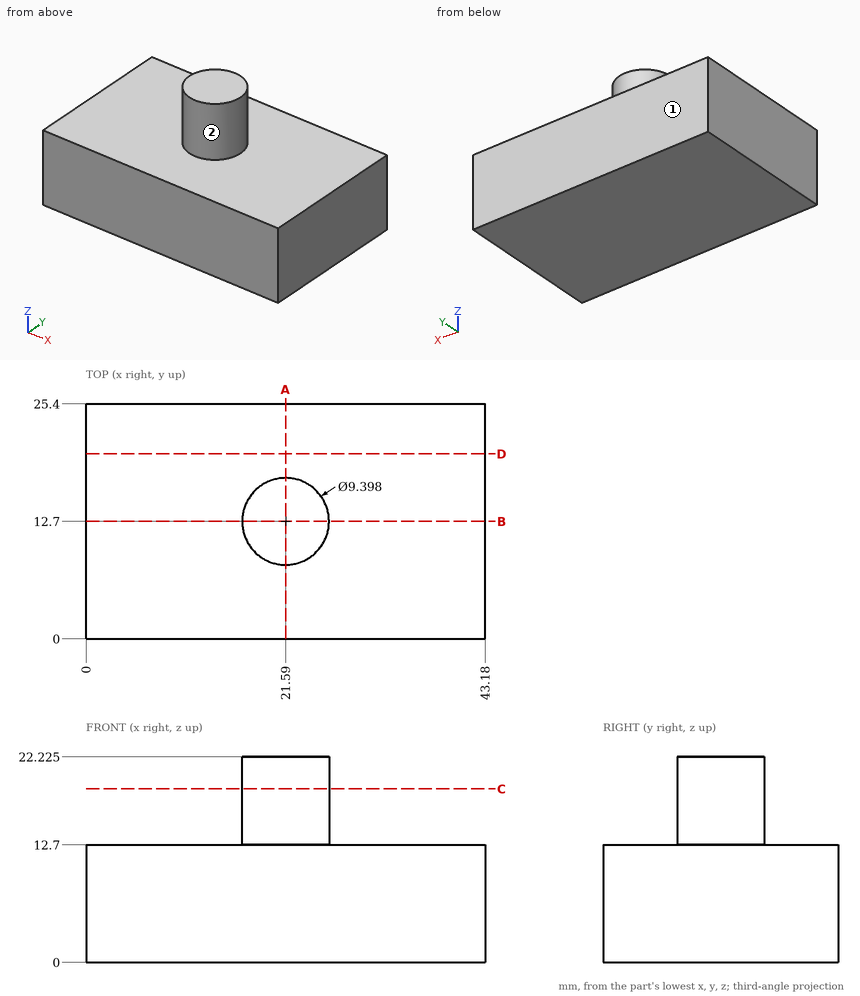
Geometry check sheet. Reference: drawing and pictorial views, mm from the part's lowest x, y, z. A direction names the side the tool comes from. Coordinates: 2 decimals unless noted, no trailing zeros. Write each loop counter-clockwise with the first axis right and the second up, starting at its lowest first coordinate (ties: lowest second). Pieces come first, ordered by that corner, then holes. Notation, with made-up numbers: M 63,-8 L 95,-8 A16 cw 95,7 Z; hole C 32,-5 d10. An arc over 180 degrees is marked long. Write item = value, one per line. Start each with the question number.
1. Thickness scan on probe 1 along Z at (x, y) = (39.5, 2.75); probe 2 along X at (y, z) = (15, 17); probe 3 along Y at (x, z) = (19, 16). Record the ranges inside material, lowest first.
2. Go/stop test with a flat-tipped pin: pin 1 (4 mm diameter, centred on x = 24.5, z = 17, fed in from +Y). Record where the tip stops, or that it passes through.
3. Sectioned sample at B-B (y = 12.7). Record the cut outline in (x, z) (3 decimals).
4. Sectioned sample at C-C (z = 18.75). Record the cut outline in (x, y), then the cut area to 3 significant figures.
5. Sectioned sample at D-D (y = 20). Record the cut outline in (x, z).
6. Tool access check on the marked faces 1 and 2. Record the directions out of +Z, -Z, +X, -X, +Y, -Y that give a thin tool (end or side, any length) a straight path to the whole face; none if there is none.
7. Sectioned sample at A-A (x = 21.59). Record the cut outline in (y, z) (3 decimals), then the cut area to 3 significant figures.
The answers:
q1.probe_1 = 0 to 12.7
q1.probe_2 = 17.49 to 25.69
q1.probe_3 = 8.78 to 16.62
q2.pin_1 = 17.31
q3.outline = M 0,0 L 43.18,0 L 43.18,12.7 L 26.289,12.7 L 26.289,22.225 L 16.891,22.225 L 16.891,12.7 L 0,12.7 Z
q4.outline = C 21.59,12.7 d9.4
q4.area = 69.4 mm²
q5.outline = M 0,0 L 43.18,0 L 43.18,12.7 L 0,12.7 Z
q6.face_1 = +Z, -Z, +X, -X, +Y
q6.face_2 = +Z
q7.outline = M 0,0 L 25.4,0 L 25.4,12.7 L 17.399,12.7 L 17.399,22.225 L 8.001,22.225 L 8.001,12.7 L 0,12.7 Z
q7.area = 412 mm²
